For this review, use the dimensioned drawing (mm, ordinates from the lowest corner) and the shaded views. A direction names the side the tool comes from. Give positions to 0.01 mm unless a question says otherwise; leave off trailing zeros. Order: outer loops, then holes, each group sorted by start corner. A loop starts at its lowest first (then second) coordinate and runs counter-clockwise, first axis right, second up. Notation, with made-up numbers: (44.5, -38) - (77.5, -38) arc R11 cw to (77.5, -24) - close; hole circle Ø1 at (25.25, 86). An arc over 180 degrees is marked (long way). One line per item, written item: value.
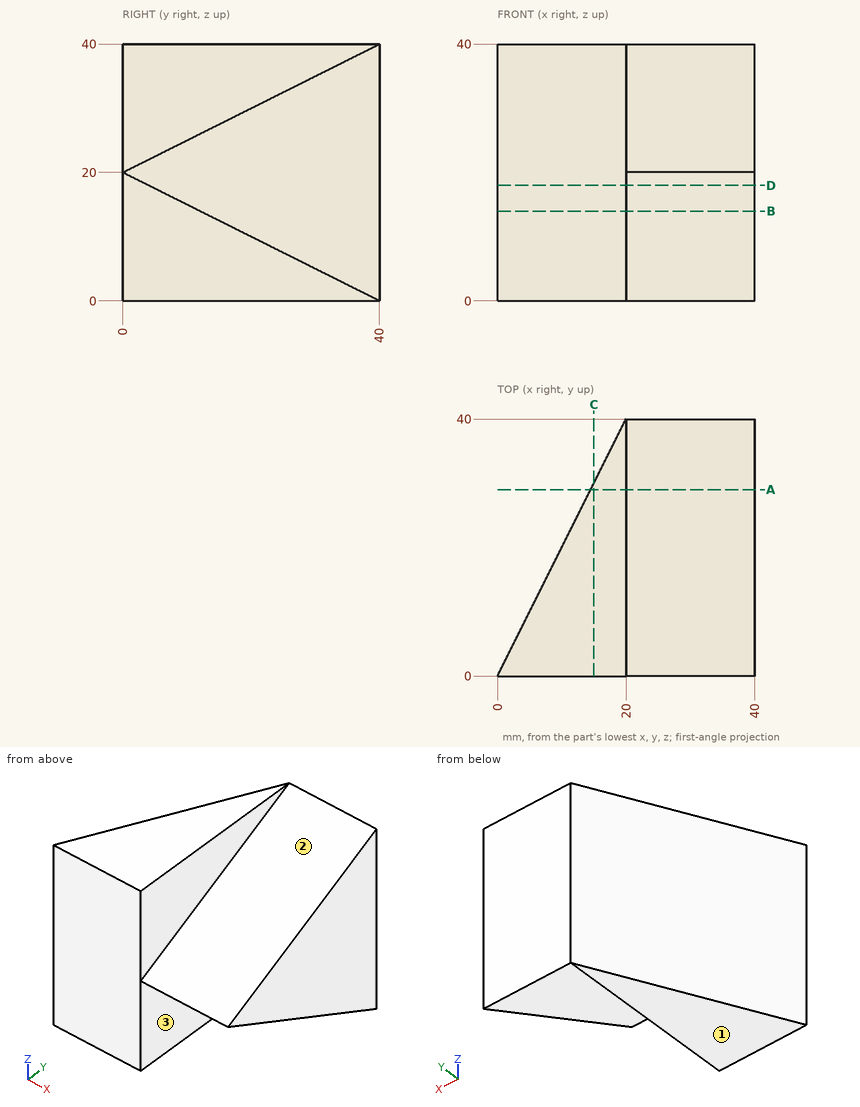
(1) Take a section at B-B (z = 14). Write out the cut boundary in (x, y).
Answers below:
outline: (0, 0) - (20, 0) - (20, 12) - (40, 12) - (40, 40) - (20, 40) - close
(2) Machinability: for the marked faces 1, 2 and 3, which of the approach directions +Z, -Z, +X, -X, +Y, -Y give a long, thin tool a straight path to every point of the face, cutting with its end or side? Answer none if there is none.
Answers below:
face 1: -Z, +X, -X, +Y, -Y
face 2: +Z, +X, -Y
face 3: -Z, +X, -Y
(3) Wall thickness on line 1 (Y direction, x = 21, z = 26.5); line 2 (X direction, y = 30, z = 12.5); line 3 (X direction, y = 16.5, z = 29): over which ranges is each line inside the solid? List them lowest first. Write a range as from..to.
Answers below:
line 1: y = 13..40
line 2: x = 15..40
line 3: x = 8.25..20
(4) Take a section at A-A (y = 29). Write out the cut boundary in (x, z), then the cut area to 3 significant figures.
Answers below:
outline: (14.5, 0) - (20, 0) - (20, 5.5) - (40, 5.5) - (40, 34.5) - (20, 34.5) - (20, 40) - (14.5, 40) - close
area: 800 mm^2
(5) For P1, Ø5, axis at y = 24.5, z = 29.5, coming from the -X side; P2, Ø10, axis at x = 27.5, y = 30, coming from the +Z side; P3, Ø2, axis at y = 4.5, z = 4.5, coming from the -X side, all flat-tipped, find the tip position at first contact; note any pin that passes through.
Answers below:
P1: stops at x = 11
P2: stops at z = 37.5
P3: stops at x = 1.75
(6) Take a section at C-C (x = 15). Write out the cut boundary in (y, z), then the cut area to 3 significant figures.
Answers below:
outline: (0, 0) - (30, 0) - (30, 40) - (0, 40) - close
area: 1,200 mm^2
(7) Take a section at D-D (z = 18). Write out the cut boundary in (x, y).
Answers below:
outline: (0, 0) - (20, 0) - (20, 4) - (40, 4) - (40, 40) - (20, 40) - close
